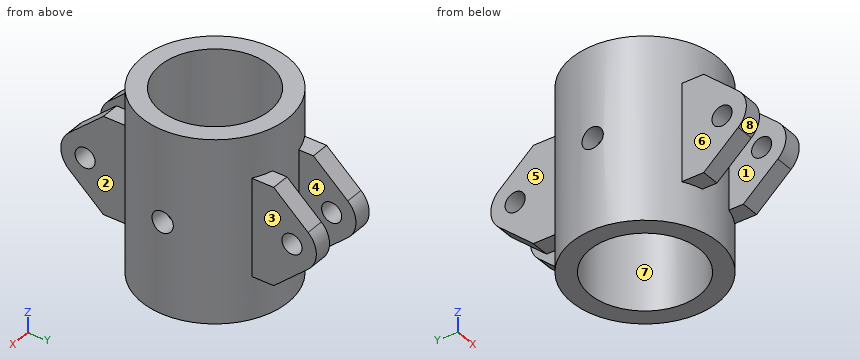
```python
from build123d import *

# Parameters (mm, degrees)
SKETCH_1_R               = 12
SKETCH_1_R_2             = 9
EXTRUDE_1_DEPTH          = 30
SKETCH_2_R               = 1.65
EXTRUDE_2_DEPTH          = 3
SKETCH_3_R               = 1.75
CUT_EXTRUDE_1_DEPTH      = 13
CUT_EXTRUDE_1_DEPTH_BACK = 13
MIRROR_2_COPY_1_SKETCH_R = 1.65
MIRROR_2_COPY_1_DEPTH    = 3


with BuildPart() as part:
    # ｽｹｯﾁ1 → ﾎﾞｽ - 押し出し1 (new body)
    with BuildSketch(Plane.XY):
        Circle(SKETCH_1_R)
        Circle(SKETCH_1_R_2, mode=Mode.SUBTRACT)
    extrude(amount=EXTRUDE_1_DEPTH)

    # ｽｹｯﾁ2 → ﾎﾞｽ - 押し出し2 (add)
    with BuildSketch(Plane(origin=(3, 0, 0), x_dir=(0, 0, -1), z_dir=(1, 0, 0))):
        with BuildLine():
            Line((-23, 9), (-23, 14))
            Line((-23, 14), (-17.994493332, 19.651982218))
            ThreePointArc((-17.994493332, 19.651982218), (-15, 21), (-12.005506668, 19.651982218))
            Line((-12.005506668, 19.651982218), (-7, 14))
            Line((-7, 14), (-7, 9))
            Line((-7, 9), (-23, 9))
        make_face()
        with Locations((-15, 17)):
            Circle(SKETCH_2_R, mode=Mode.SUBTRACT)
    extrude_2 = extrude(amount=EXTRUDE_2_DEPTH)

    # ﾐﾗｰ1: ﾎﾞｽ - 押し出し2 across plane
    add(extrude_2.mirror(Plane(origin=(0, 0, 0), x_dir=(0, 0, 1), z_dir=(1, 0, 0))))

    # ｽｹｯﾁ3 → ｶｯﾄ - 押し出し1 (cut, two sides)
    with BuildSketch(Plane(origin=(0, 0, 0), x_dir=(0, 0, -1), z_dir=(1, 0, 0))) as cut_extrude_1_sk:
        with Locations((-15, 0)):
            Circle(SKETCH_3_R)
    extrude(amount=CUT_EXTRUDE_1_DEPTH, mode=Mode.SUBTRACT)
    extrude(cut_extrude_1_sk.sketch, amount=-CUT_EXTRUDE_1_DEPTH_BACK, mode=Mode.SUBTRACT)

    # ﾐﾗｰ2: ﾎﾞｽ - 押し出し2 across plane
    add(extrude_2.mirror(Plane.ZX))

    # ﾐﾗｰ2 copy 1 sketch → ﾐﾗｰ2 copy 1 (add)
    with BuildSketch(Plane(origin=(-3, 0, 0), x_dir=(0, 0, -1), z_dir=(-1, 0, 0))):
        with BuildLine():
            Line((-23, 9), (-23, 14))
            Line((-23, 14), (-17.994493332, 19.651982218))
            ThreePointArc((-17.994493332, 19.651982218), (-15, 21), (-12.005506668, 19.651982218))
            Line((-12.005506668, 19.651982218), (-7, 14))
            Line((-7, 14), (-7, 9))
            Line((-7, 9), (-23, 9))
        make_face()
        with Locations((-15, 17)):
            Circle(MIRROR_2_COPY_1_SKETCH_R, mode=Mode.SUBTRACT)
    extrude(amount=MIRROR_2_COPY_1_DEPTH)


solid = part.part
```
Part model, mm, in its own coordinate system. Face numbers are marked on the shaded views. A direction names the side the tool comes from. Give positions to 0.01 mm unless a question says otherwise; leave off trailing zeros. Write each loop counter-clockwise with the first axis right and the second up, starting at its lowest first coordinate (ties: lowest second). Pieces come first, ordered by that corner, then holes. Notation, with made-up numbers: (61.5, -7.75) -> (65.5, -7.75) arc R20 ccw to (65.5, 10.25) -> close; hole circle Ø3 at (-3, -35.5). An arc over 180 degrees is marked (long way). Put each result on its own line as item: value. Start each with the question number.
Item 1: Cut at A-A (y = 0). List the corners of the cut face in (x, z).
Item 2: Pull direction Y, two halves, no side cores. Call the marked faces 6, 7 and 8: pulls with the +Y half, pulls with the -Y half, needs draft (parallel to the pull), parting line crosses it, or undercut.
Item 3: Cut at B-B (x = 0). List the corners of the cut face in (y, z).
Item 4: Pin check, flat tips, straight feed: pin 1 Ø0.9 at (x, y) = (-4.5, -13) entering from -Z; pin 2 Ø7.5 at (y, z) = (18, 17) entering from -X; pin 3 Ø12 at (x, y) = (-5.5, -7) entering from +Z; pin 4 Ø8 at (y, z) = (-4.5, 15.5) entering from +X. Stop position of each tip, or through.
Item 5: Cut at C-C (z = 20.5). List the corners of the cut face in (x, y).
Item 6: Which spindle directions (+Z, -Z, +X, -X, +Y, -Y) get a long thin tool onto all of the face, cutting with end or side? Do the marked faces 1, 2, 3, 4 and 5. Say none if no direction does.
Item 7: Wall check: L1, parallel to Y at x = 4, z = 15; L2, parallel to X at y = 0, z = 22; L3, parallel to Y at x = -4.4, z = 15. Give the ranges that are in metal, low to high. Write a range as [from, to].
Item 8: Cut at D-D (y = 5.5). List the corners of the cut face in (x, z).
Answer list:
1. outline: (-12, 0) -> (-9, 0) -> (-9, 13.25) -> (-12, 13.25) -> close; (-12, 16.75) -> (-9, 16.75) -> (-9, 30) -> (-12, 30) -> close; (9, 0) -> (12, 0) -> (12, 13.25) -> (9, 13.25) -> close; (9, 16.75) -> (12, 16.75) -> (12, 30) -> (9, 30) -> close
2. face 6: needs draft
2. face 7: undercut
2. face 8: pulls with the -Y half
3. outline: (-12, 0) -> (-9, 0) -> (-9, 30) -> (-12, 30) -> close; (9, 0) -> (12, 0) -> (12, 30) -> (9, 30) -> close
4. pin 1: stops at z = 7
4. pin 2: stops at x = -6
4. pin 3: stops at z = 30
4. pin 4: stops at x = 11.98
5. outline: (-6, -16.82) -> (-3, -16.82) -> (-3, -11.62) arc R12 ccw to (3, -11.62) -> (3, -16.82) -> (6, -16.82) -> (6, -10.39) arc R12 ccw to (6, 10.39) -> (6, 16.82) -> (3, 16.82) -> (3, 11.62) arc R12 ccw to (-3, 11.62) -> (-3, 16.82) -> (-6, 16.82) -> (-6, 10.39) arc R12 ccw to (-6, -10.39) -> close; hole circle Ø18 at (0, 0)
6. face 1: +Z, -Z, -Y
6. face 2: +Z, -Z, +X, -Y
6. face 3: +Z, -Z, +X, +Y
6. face 4: +Z, -Z, +Y
6. face 5: +Z, -Z, -X, +Y
7. L1: y = [-21, -18.65], [-15.35, -8.06], [8.06, 15.35], [18.65, 21]
7. L2: x = [-12, -9], [9, 12]
7. L3: y = [-21, -18.65], [-15.35, -7.85], [7.85, 15.35], [18.65, 21]
8. outline: (-10.67, 0) -> (-7.12, 0) -> (-7.12, 30) -> (-10.67, 30) -> close; (7.12, 0) -> (10.67, 0) -> (10.67, 30) -> (7.12, 30) -> close
